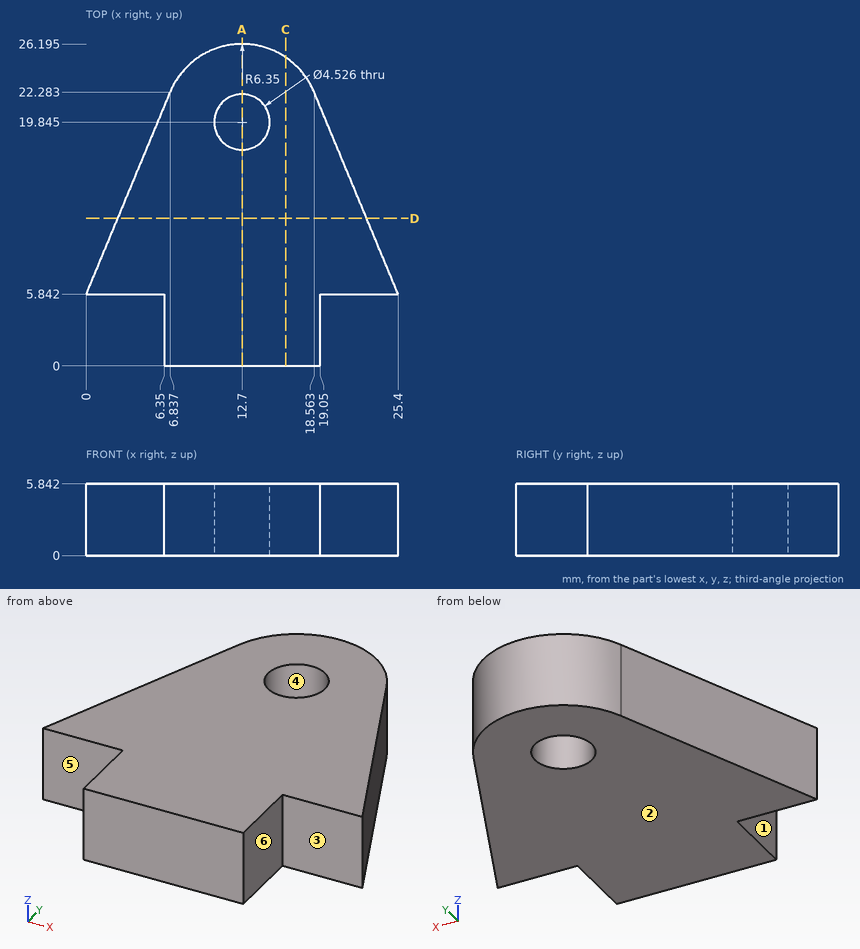
Verification items for this drawing (mm, ordinates from the low corner). A direction names the side the tool comes from. Coordinates: 2 decimals unless noted, no trailing zeros. Loops run counter-clockwise (first coordinate to the right, second up) from the corner with the lowest first, then second, coordinate; pieces in that order, holes last.
Item 1: Sectioned sample at D-D, the plane y = 12. Record the boundary of the cut face in (x, z).
Item 2: Go/stop test with flat-tipped pins: pin 1 Ø1 at (y, z) = (7, 4.5) entering from +X; pin 2 Ø1.8 at (x, z) = (4.5, 2) entering from -Y; pin 3 Ø3 at (y, z) = (1.5, 3.5) entering from +X. Record where each tip stops, or that it passes through.
Item 3: Sectioned sample at C-C, the plane x = 16.25. Record the boundary of the cut face in (y, z), then the cut area to 3 significant figures.
Item 4: Release check for a two-part mould opening along X. For the marked faces 4, 5 and 6 record: released by +X, released by -X, zero draft, split by the parting line, or undercut.
Item 5: Sectioned sample at A-A, the plane x = 12.7. Record the boundary of the cut face in (y, z) (1 decimal).
Item 6: Thickness scan on line 1 (Y direction, x = 12.7, z = 1.7) (1 decimal); line 2 (X direction, y = 1, z = 1.25); line 3 (X direction, y = 21.75, z = 2.05) (1 decimal). Record the ranges inside material, lowest first.
Item 7: Access from +Z, -Z, +X, -X, +Y, -Y to the whole of each face (thin tool, end or side, straight path). Record for the marked faces 1, 2 and 3.
Check result:
1. outline: (2.56, 0) - (22.84, 0) - (22.84, 5.84) - (2.56, 5.84) - close
2. pin 1: stops at x = 25.13
2. pin 2: stops at y = 5.84
2. pin 3: stops at x = 19.05
3. outline: (0, 0) - (25.11, 0) - (25.11, 5.84) - (0, 5.84) - close
3. area: 147 mm2
4. face 4: undercut
4. face 5: zero draft
4. face 6: released by +X
5. outline: (0, 0) - (17.6, 0) - (17.6, 5.8) - (0, 5.8) - close; (22.1, 0) - (26.2, 0) - (26.2, 5.8) - (22.1, 5.8) - close
6. line 1: y = 0 to 17.6, 22.1 to 26.2
6. line 2: x = 6.35 to 19.05
6. line 3: x = 6.6 to 11.5, 13.9 to 18.8
7. face 1: +Z, -Z, -X, -Y
7. face 2: -Z, +X, -X, +Y, -Y
7. face 3: +Z, -Z, +X, -Y
